The listing builds one solid part. Answer for the finished solid, in the listing's coordinates (mm). A direction names the side the tool comes from. Coordinates: 2 decimals unless noted, no trailing zeros. Loops run counter-clockwise (first coordinate to the right, second up) from the corner with the lowest first, then second, coordinate; pieces in that order, holes last. Notation, with made-up numbers: M 53.5,34.25 L 73.5,34.25 A6 cw 73.5,42.25 Z; hole C 84.5,61 d2. An arc over 180 degrees is marked long. Return JSON: item names as keys, results as strings. Group by question number.
1. The mould has two halves that part along Y. Classify faces 3 (the face through (0, 8, 2)), 4 (the face through (-19.474, 3.755, -11.923)), 5 (the face through (-37.528, 3.584, -2.285)), 6 (the face through (-18, -10, 0)): pulls with the +Y half, pulls with the -Y half, needs draft (parallel to the pull), parting line crosses it, or undercut.
2. Section B-B (y = 0) is taken. Write down the section's boundary in (x, z).
3. Section C-C (x = -17) is taken. Write down the section's boundary in (y, z), then the cut area to 3 significant figures.
4. Straight lines are drawn through the part: L1, parallel to Y at x = -27.5, z = 0; L2, parallel to Y at x = -37.75, z = 0; L3, parallel to Z at x = -14.5, y = 8. For each, find the intervals that lie inside material, in ascending order. Write a range as from..to.
5. Section A-A (z = 0) is taken. Write down the section's boundary in (x, y).
6. Given P1, Ø1.1, axis at x = -18, y = 8.5, coming from the +Z side; P2, Ø1.5, axis at x = -5, z = -6.5, coming from the -Y side; P3, Ø8, axis at x = -8, z = -4, coming from the +Y side; P4, Ø2, axis at y = 4.5, z = 5.5, coming from the +X side, each flat-ended and moving along its own axis, determine where each tip first touches the part or whether it passes through.
7. Which of the six approach directions +Z, -Z, +X, -X, +Y, -Y give full straight-line access (tool end or side, diameter ignored) to faces 1 (the face through (-39.5, -5, 0)), 2 (the face through (-18, 9, -2.5))?
8. Section D-D (y = -6) is taken. Write down the section's boundary in (x, z).
```python
from build123d import *

# Parameters (mm, degrees)
SKETCH_2_W      = 5
SKETCH_2_H      = 2.5
EXTRUDE_1_DEPTH = 39.5


with BuildPart() as part:
    # Эскиз1 → Повернуть1 (revolve)
    with BuildSketch(Plane(origin=(0, 0, 0), x_dir=(1, 0, 0), z_dir=(0, 1, 0))):
        Polygon((0, 10), (-35.5, 10), (-35.5, 4.25), (-39.5, 4.25), (-39.5, 12.5), (0, 12.5), align=None)
    revolve(axis=Axis((-1000, 0, 0), (1, 0, 0)))

    # Эскиз2 → Бобышка-Вытянуть1 (add)
    with BuildSketch(Plane.ZY.offset(39.5)):
        with Locations((0, 8.75)):
            Rectangle(SKETCH_2_W, SKETCH_2_H)
    extrude(amount=-EXTRUDE_1_DEPTH)


solid = part.part
```
Worked out:
{
 "1": {"face 3": "needs draft", "face 4": "parting line crosses it", "face 5": "undercut", "face 6": "undercut"},
 "2": {"outline": "M -39.5,-12.5 L 0,-12.5 L 0,-10 L -35.5,-10 L -35.5,-4.25 L -39.5,-4.25 Z; M -39.5,4.25 L -35.5,4.25 L -35.5,10 L 0,10 L 0,12.5 L -39.5,12.5 Z"},
 "3": {"outline": "C 0,0 d25; hole M 7.5,-2.5 L 7.5,2.5 L 9.68,2.5 A10 ccw long 9.68,-2.5 Z", "area": "189 mm^2"},
 "4": {"L1": "-12.5..-10, 7.5..12.5", "L2": "-12.5..-4.25, 4.25..12.5", "L3": "-9.6..-6, -2.5..2.5, 6..9.6"},
 "5": {"outline": "M -39.5,-12.5 L 0,-12.5 L 0,-10 L -35.5,-10 L -35.5,-4.25 L -39.5,-4.25 Z; M -39.5,4.25 L -35.5,4.25 L -35.5,7.5 L 0,7.5 L 0,12.5 L -39.5,12.5 Z"},
 "6": {"P1": "z = 9.65", "P2": "y = -11.1", "P3": "y = 12.5", "P4": "x = -35.5"},
 "7": {"face 1": "+Z, -Z, -X, +Y, -Y", "face 2": "+X"},
 "8": {"outline": "M -39.5,-10.97 L 0,-10.97 L 0,-8 L -35.5,-8 L -35.5,8 L 0,8 L 0,10.97 L -39.5,10.97 Z"}
}
